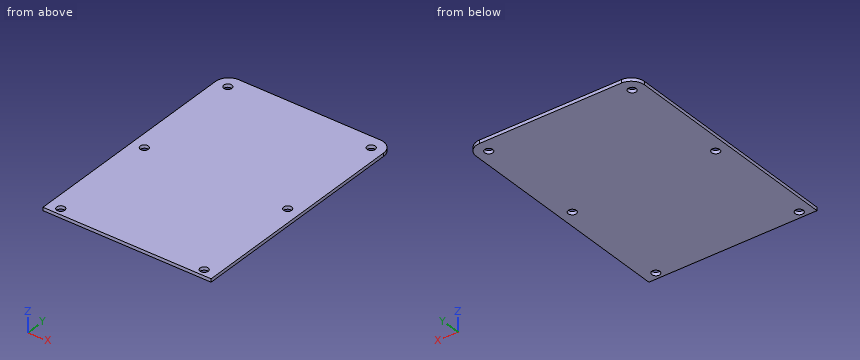
```python
from build123d import *

# Parameters (mm, degrees)
EXTRUDE_1_DEPTH     = 0.8
SKETCH_2_R          = 1
CUT_EXTRUDE_1_DEPTH = 81.091837911


with BuildPart() as part:
    # 草图1 → 凸台-拉伸1 (new body)
    with BuildSketch(Plane.XY):
        with BuildLine():
            Line((-41.75, 66.25), (-6.75, 66.25))
            ThreePointArc((-6.75, 66.25), (-4.451902961, 65.298097039), (-3.5, 63))
            Line((-3.5, 63), (-3.5, 7.25))
            Line((-3.5, 7.25), (-45, 7.25))
            Line((-45, 7.25), (-45, 63))
            ThreePointArc((-45, 63), (-44.048097039, 65.298097039), (-41.75, 66.25))
        make_face()
    extrude(amount=EXTRUDE_1_DEPTH)

    # 草图2 → 切除-拉伸1 (cut, through all)
    with BuildSketch(Plane.XY.offset(0.8)):
        with Locations((-41.95, 63)):
            Circle(SKETCH_2_R)
        with Locations((-41.95, 36)):
            Circle(SKETCH_2_R)
        with Locations((-41.95, 9)):
            Circle(SKETCH_2_R)
        with Locations(Location((-6.55, 9, 0), (0, 0, 180))):
            Circle(SKETCH_2_R)
        with Locations(Location((-6.55, 36, 0), (0, 0, 180))):
            Circle(SKETCH_2_R)
        with Locations(Location((-6.55, 63, 0), (0, 0, 180))):
            Circle(SKETCH_2_R)
    extrude(amount=-CUT_EXTRUDE_1_DEPTH, mode=Mode.SUBTRACT)


solid = part.part
```
Part model, mm, in its own coordinate system. Give positions to 0.01 mm unless a question says otherwise; leave off trailing zeros. Loops run counter-clockwise (first coordinate to the right, second up) from the corner with the lowest first, then second, coordinate; pieces in that order, holes last. Notation, with made-up numbers: M -37,69 L 8,69 A19 cw 8,79 Z; hole C 30,17.25 d3. An arc over 180 degrees is marked long. Return JSON: item names as keys, results as strings.
1) Drill centre line: line 1 (Y direction, x = -6.55, z = 0.2). Where is it in solid material? Low to high.
Calculated:
{"line 1": "y = 7.25 to 8, 10 to 35, 37 to 62, 64 to 66.24"}
2) Saw through at A-A, the plane y = 9. List the corners of the cut face in (x, z), then the cut area to 3 significant figures.
Calculated:
{"outline": "M -45,0 L -42.95,0 L -42.95,0.8 L -45,0.8 Z; M -40.95,0 L -7.55,0 L -7.55,0.8 L -40.95,0.8 Z; M -5.55,0 L -3.5,0 L -3.5,0.8 L -5.55,0.8 Z", "area": "30.0 mm2"}
3) Flat gauge pins, fed straight in: pin 1 Ø1.8 at (x, y) = (-41.95, 36) entering from +Z; pin 2 Ø3 at (x, y) = (-6.55, 9) entering from -Z. Where does each tip first touch, or does it go through?
Calculated:
{"pin 1": "passes through", "pin 2": "stops at z = 0"}
